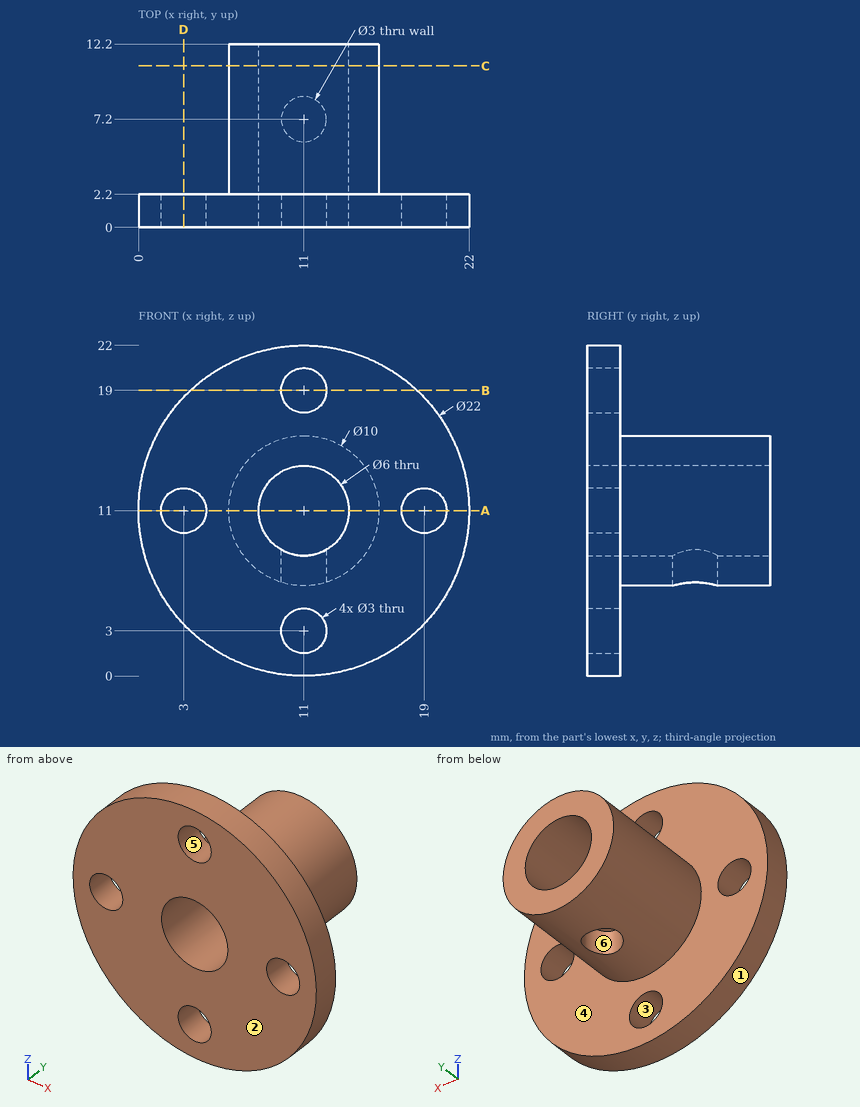
Here's the drawing with two shaded views (mm, measured from the low corner). I have some questions. A direction names the side the tool comes from. Give positions to 0.01 mm unless a question says otherwise; leave off trailing zeros. Order: outer loops, then holes, each group sorted by start corner. A loop starts at its lowest first (then second) coordinate and runs counter-clockwise, first axis right, second up. Notation, with made-up numbers: M -31,39 L 17,39 A17 cw 17,54 Z; hole C -25.5,-34 d8. An arc over 180 degrees is marked long. One line per question, with ' | ' between items.
Item 1: We'd pull the mould along Z, two halves only. Please class the marked faces 1, 2 and 3: released by +Z, released by -Z, zero draft, split by the parting line, or undercut.
Answer block:
face 1: split by the parting line | face 2: zero draft | face 3: undercut
Item 2: Suppose I cut it at B-B, the plane z = 19. Write out the boundary of the cut face in (x, y), then the cut area to 3 significant figures.
Answer block:
outline: M 3.45,0 L 9.5,0 L 9.5,2.2 L 3.45,2.2 Z; M 12.5,0 L 18.55,0 L 18.55,2.2 L 12.5,2.2 Z | area: 26.6 mm2
Item 3: I'm going to push flat-ended pins straight in: pin 1 Ø2 at (x, z) = (17.5, 12.5) entering from +Y; pin 2 Ø1.5 at (y, z) = (4, 16) entering from +X; pin 3 Ø6 at (x, y) = (7.5, 10.5) entering from +Z. Where does each tip first touch, or does it pass through?
Answer block:
pin 1: stops at y = 2.2 | pin 2: stops at x = 13.63 | pin 3: stops at z = 15.97
Item 4: Suppose I cut it at D-D, the plane x = 3. Write out the boundary of the cut face in (y, z), then the cut area to 3 significant figures.
Answer block:
outline: M 0,3.45 L 2.2,3.45 L 2.2,9.5 L 0,9.5 Z; M 0,12.5 L 2.2,12.5 L 2.2,18.55 L 0,18.55 Z | area: 26.6 mm2
Item 5: Suppose I cut it at C-C, the plane y = 10.75. Write out the boundary of the cut face in (x, z), then the cut area to 3 significant figures.
Answer block:
outline: C 11,11 d10; hole C 11,11 d6 | area: 50.3 mm2
Item 6: For the marked faces 4, 5 and 6, which set-ups out of +Z, -Z, +X, -X, +Y, -Y let a thin tool reach every point of the face, with its end or its side?
Answer block:
face 4: +Y | face 5: +Y, -Y | face 6: -Z
Item 7: Suppose I cut it at A-A, the plane z = 11. Write out the boundary of the cut face in (x, y).
Answer block:
outline: M 0,0 L 1.5,0 L 1.5,2.2 L 0,2.2 Z; M 4.5,0 L 8,0 L 8,12.2 L 6,12.2 L 6,2.2 L 4.5,2.2 Z; M 14,0 L 17.5,0 L 17.5,2.2 L 16,2.2 L 16,12.2 L 14,12.2 Z; M 20.5,0 L 22,0 L 22,2.2 L 20.5,2.2 Z
Item 8: Please list where these lines run through material, in increasing order: L1, parallel to X at y = 0.5, z = 11; L2, parallel to Y at x = 17.75, z = 4; L3, parallel to X at y = 2.75, z = 11.
Answer block:
L1: x = 0 to 1.5, 4.5 to 8, 14 to 17.5, 20.5 to 22 | L2: y = 0 to 2.2 | L3: x = 6 to 8, 14 to 16
